Design review of the part shown in the three views and the two pictorial views. Dimensions are in mm from the part's minimum x, y and z. A direction names the side the tool comes from. Give positions to 0.01 mm unless a question says otherwise; leave off trailing zeros. Write each loop counter-clockwise with the first axis right and the second up, starting at its lowest first coordinate (ties: lowest second). Pieces come first, ordered by that corner, then holes. Notation, with made-up numbers: M 45,80.25 L 78,80.25 A25 cw 78,92.25 Z; hole C 21.25,-25 d10. An arc over 180 degrees is marked long. Write item = value, one per line.
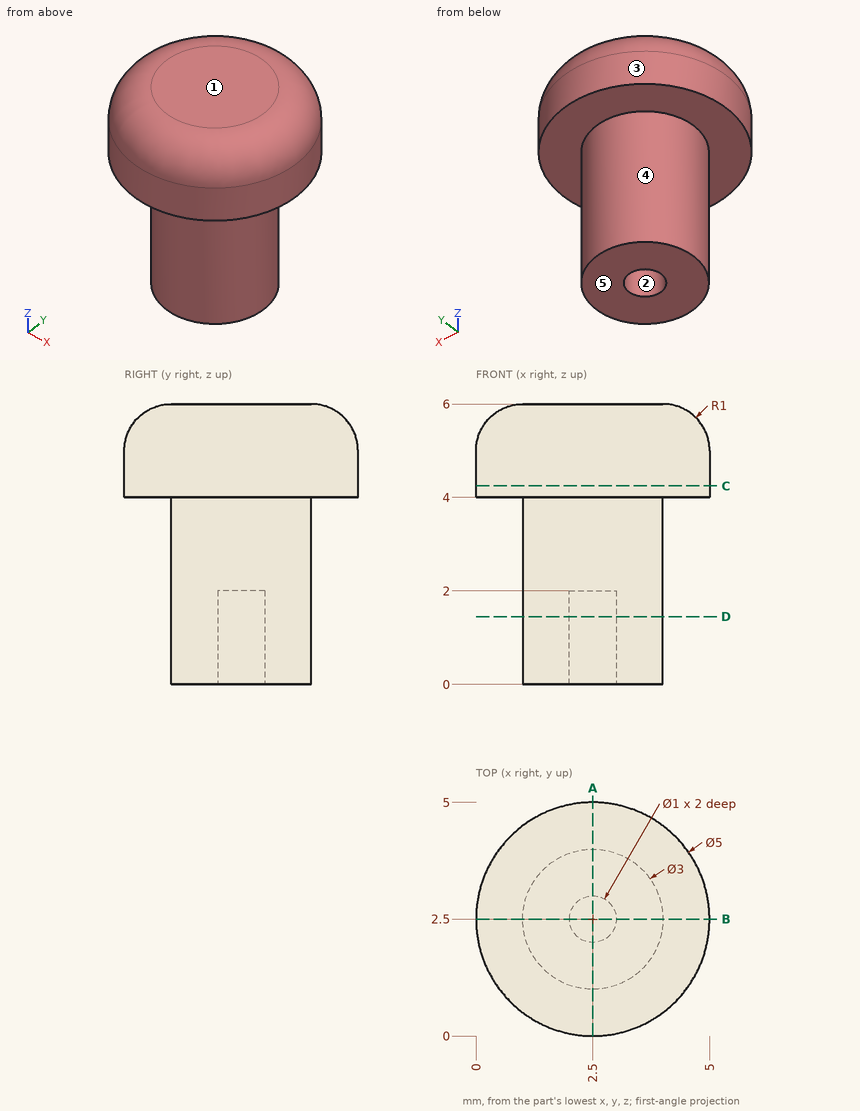
1. Insertion check: P1, Ø2.5, axis at x = 3.5, y = 2.5, coming from the -Z side. The pin has a flat end and moves straight along its axis. Give the tip position at first contact, or say it passes through.
Responses:
P1 = 0
2. We need section D-D, the plane z = 1.45. Write out the cut boundary in (x, y), then the cut area to 3 significant figures.
Responses:
outline = C 2.5,2.5 d3; hole C 2.5,2.5 d1
area = 6.28 mm2
3. For line 1 along Y through (x, z) = (2.5, 0.9); line 2 along Z through (x, y) = (2.9, 2.65); line 3 along Z through (x, y) = (4.65, 3.5), list the stretches that pass through material, from the lowest coordinate up. Write a range as from..to.
Responses:
line_1 = 1..2, 3..4
line_2 = 2..6
line_3 = 4..5.49
4. We need section A-A, the plane x = 2.5. Write out the cut boundary in (y, z).
Responses:
outline = M 0,4 L 1,4 L 1,0 L 2,0 L 2,2 L 3,2 L 3,0 L 4,0 L 4,4 L 5,4 L 5,5 A1 ccw 4,6 L 1,6 A1 ccw 0,5 Z
5. The part is to be moulded in two halves that separate along Y. For the marked faces 1, 2 and 3, say which applies: +Y half, -Y half, draft (parallel to the pull), parting line (faces both ways), or undercut.
Responses:
face_1 = draft
face_2 = undercut
face_3 = parting line
6. We need section C-C, the plane z = 4.25. Write out the cut boundary in (x, y), then the cut area to 3 significant figures.
Responses:
outline = C 2.5,2.5 d5
area = 19.6 mm2
7. Machinability: for the marked faces 4 and 5, which of the approach directions +Z, -Z, +X, -X, +Y, -Y give a long, thin tool a straight path to every point of the face, cutting with its end or side? Answer none if there is none.
Responses:
face_4 = -Z
face_5 = -Z, +X, -X, +Y, -Y
